```python
from build123d import *

# Parameters (mm, degrees)
SKETCH_2_W           = 60
SKETCH_2_H           = 60
EXTRUDE_1_DEPTH      = 7
EXTRUDE_2_DEPTH      = 11.5
EXTRUDE_2_DEPTH_BACK = 11.5


with BuildPart() as part:
    # 草图2 → 凸台-拉伸1 (new body)
    with BuildSketch(Plane(origin=(0, 0, 0), x_dir=(1, 0, 0), z_dir=(0, 1, 0))):
        Rectangle(SKETCH_2_W, SKETCH_2_H)
    extrude(amount=EXTRUDE_1_DEPTH)

    # 草图3 → 凸台-拉伸2 (add, two sides: drawn at the far end of the back side and taken through both)
    with BuildSketch(Plane.XY.offset(-EXTRUDE_2_DEPTH_BACK)):
        with BuildLine():
            Line((-28.405989232, 58.5), (28.405989232, 58.5))
            Line((28.405989232, 58.5), (28.405989232, 66.5))
            Line((28.405989232, 66.5), (28.405989232, 106.5))
            Line((28.405989232, 106.5), (51.5, 66.5))
            Line((51.5, 66.5), (51.5, 58.5))
            ThreePointArc((51.5, 58.5), (41.38085306, 27.842619159), (15, 9.232870999))
            Line((15, 9.232870999), (15, 7))
            Line((15, 7), (-15, 7))
            Line((-15, 7), (-15, 9.232870999))
            ThreePointArc((-15, 9.232870999), (-41.38085306, 27.842619159), (-51.5, 58.5))
            Line((-51.5, 58.5), (-51.5, 66.5))
            Line((-51.5, 66.5), (-28.405989232, 106.5))
            Line((-28.405989232, 106.5), (-28.405989232, 66.5))
            Line((-28.405989232, 66.5), (-28.405989232, 58.5))
        make_face()
    extrude(amount=EXTRUDE_2_DEPTH + EXTRUDE_2_DEPTH_BACK)


solid = part.part
```
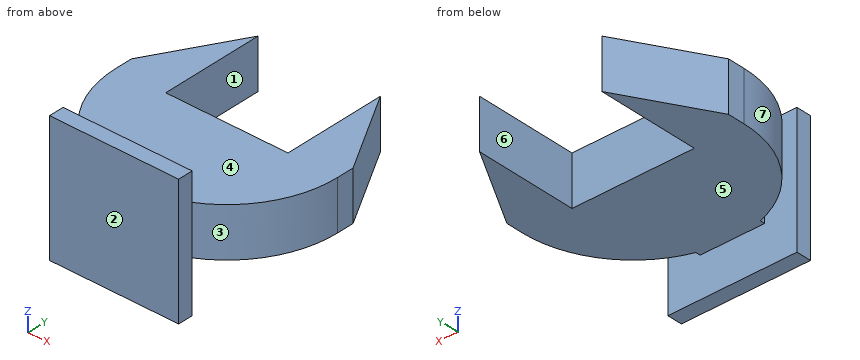
Build history of the part. All positions in model axes, mm. Face numbers are marked on the shaded views. A direction names the side the tool comes from. Round coordinates to 2 decimals unless told otherwise and drop trailing zeros. Write each loop counter-clockwise with the first axis right and the second up, starting at its lowest first coordinate (ties: lowest second). Pieces come first, ordered by that corner, then holes. Notation, with made-up numbers: (-29.5, 67.25) - (13.5, 67.25) arc R20 ccw to (13.5, 95.25) - close; hole circle Ø11 at (-22.5, 54). An arc over 180 degrees is marked (long way). Write each question's results on one line, items separated by ' | '. Start each with the question number.
Item 1: Saw through at C-C (y = 88.5). Write the cut outline in (x, z), and give its area (3 significant figures).
Item 2: Saw through at B-B (z = -3). Write the cut outline in (x, y).
Item 3: Wall check: L1, parallel to Y at x = -5.5, z = -26.5; L2, parallel to X at y = 73, z = 9.5; L3, parallel to X at y = 74, z = -4. Give the ranges that are in metal, low to high. Write a range as [from, to].
Item 4: Which spindle directions (+Z, -Z, +X, -X, +Y, -Y) get a long thin tool onto all of the face, cutting with end or side? Do the marked faces 4, 5, 6 and 7. Say none if no direction does.
Item 5: Saw through at A-A (x = -26.5). Write the cut outline in (y, z).
Item 6: Saw through at D-D (x = -7.5). Write the cut outline in (y, z), and give its area (3 significant figures).
Item 7: Mould opens along Y. For the marked faces 1, 2 and 3 say: pulls with the +Y half, pulls with the -Y half, needs draft (parallel to the pull), parting line crosses it, or undercut.
Item 8: Drop flat-ended pins along their axis: P1, Ø7, axis at y = 82, z = 0.5, coming from the -X side; P2, Ø0.7, axis at y = 7.5, z = 2, coming from the -X side; P3, Ø5.5, axis at y = 5, z = 13.5, coming from the +X side; P4, Ø6, axis at y = 32.5, z = 15, coming from the -X side. Give the stop position or say it passes through.
Results are:
1) outline: (-38.8, -11.5) - (-28.41, -11.5) - (-28.41, 11.5) - (-38.8, 11.5) - close; (28.41, -11.5) - (38.8, -11.5) - (38.8, 11.5) - (28.41, 11.5) - close | area: 478 mm²
2) outline: (-51.5, 58.5) arc R51.5 ccw to (-15, 9.23) - (-15, 7) - (-30, 7) - (-30, 0) - (30, 0) - (30, 7) - (15, 7) - (15, 9.23) arc R51.5 ccw to (51.5, 58.5) - (51.5, 66.5) - (28.41, 106.5) - (28.41, 58.5) - (-28.41, 58.5) - (-28.41, 106.5) - (-51.5, 66.5) - close
3) L1: y = [0, 7] | L2: x = [-47.75, -28.41], [28.41, 47.75] | L3: x = [-47.17, -28.41], [28.41, 47.17]
4) face 4: +Z, +X, -X, +Y | face 5: -Z, +X, -X, +Y | face 6: +Z, -Z, +Y | face 7: +Z, -Z, -X
5) outline: (0, -30) - (7, -30) - (7, 30) - (0, 30) - close; (14.34, -11.5) - (58.5, -11.5) - (58.5, 11.5) - (14.34, 11.5) - close
6) outline: (0, -30) - (7, -30) - (7, -11.5) - (58.5, -11.5) - (58.5, 11.5) - (7, 11.5) - (7, 30) - (0, 30) - close | area: 1,600 mm²
7) face 1: needs draft | face 2: pulls with the -Y half | face 3: undercut
8) P1: stops at x = -44.57 | P2: stops at x = -15 | P3: stops at x = 30 | P4: passes through
